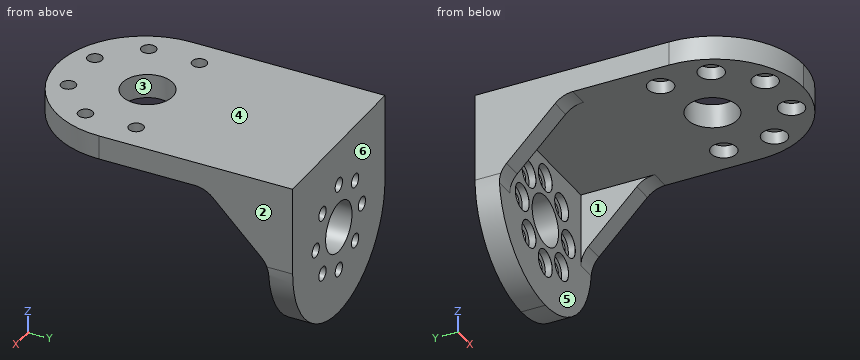
```python
from build123d import *

# Parameters (mm, degrees)
SKETCH1_W                      = 70
SKETCH1_H                      = 70
BOSS_EXTRUDE1_DEPTH            = 9.525
CBORE_FOR_M5_SBHCS1_AT_2_COUNT = 2
CBORE_FOR_M5_SBHCS1_AT_2_PITCH = 13.393920133
CBORE_FOR_M5_SBHCS1_AT_3_COUNT = 2
CBORE_FOR_M5_SBHCS1_AT_3_PITCH = 24.748737342
CBORE_FOR_M5_SBHCS1_AT_4_COUNT = 2
CBORE_FOR_M5_SBHCS1_AT_4_PITCH = 32.335783638
CBORE_FOR_M5_SBHCS1_AT_5_COUNT = 2
CBORE_FOR_M5_SBHCS1_AT_5_PITCH = 35
CBORE_FOR_M5_SBHCS1_AT_6_COUNT = 2
CBORE_FOR_M5_SBHCS1_AT_6_PITCH = 32.335783638
CBORE_FOR_M5_SBHCS1_AT_7_COUNT = 2
CBORE_FOR_M5_SBHCS1_AT_7_PITCH = 24.748737342
CBORE_FOR_M5_SBHCS1_AT_8_COUNT = 2
CBORE_FOR_M5_SBHCS1_AT_8_PITCH = 13.393920133
SKETCH5_R                      = 10
CUT_EXTRUDE1_DEPTH             = 51.405611047
SKETCH6_W                      = 70
SKETCH6_H                      = 102
BOSS_EXTRUDE2_DEPTH            = 9.525
CBORE_FOR_M5_SHCS1_D           = 5.8
CBORE_FOR_M5_SHCS1_CBORE_D     = 10
CBORE_FOR_M5_SHCS1_CBORE_DEPTH = 5
SKETCH7_R                      = 10
CUT_EXTRUDE3_DEPTH             = 9.525
BOSS_EXTRUDE3_DEPTH            = 8
FILLET1_R                      = 10
FILLET1_OF_MIRROR1_R           = 10
FILLET2_R                      = 35


with BuildPart() as part:
    # Sketch1 → Boss-Extrude1 (new body)
    with BuildSketch(Plane(origin=(0, 0, 0), x_dir=(1, 0, 0), z_dir=(0, 1, 0))):
        Rectangle(SKETCH1_W, SKETCH1_H)
    extrude(amount=BOSS_EXTRUDE1_DEPTH)

    # Sketch4 → CBORE for M5 SBHCS1 (revolve, cut)
    with BuildSketch(Plane(origin=(17.5, 0, 0), x_dir=(0, 0, -1), z_dir=(1, 0, 0))):
        Polygon((0, 0), (0, 9.525), (2.75, 9.525), (2.75, 2.75), (5.25, 2.75), (5.25, 0.025), (5.275, 0), align=None)
    cbore_for_m5_sbhcs1 = revolve(axis=Axis((17.5, -6.35, 0), (0, 1, 0)), mode=Mode.SUBTRACT)

    # CBORE for M5 SBHCS1 at 2: CBORE for M5 SBHCS1 ×2
    with Locations(*[Vector(-0.3826834323650897, 0, -0.9238795325112868) * (i * CBORE_FOR_M5_SBHCS1_AT_2_PITCH) for i in range(1, CBORE_FOR_M5_SBHCS1_AT_2_COUNT)]):
        add(cbore_for_m5_sbhcs1, mode=Mode.SUBTRACT)

    # CBORE for M5 SBHCS1 at 3: CBORE for M5 SBHCS1 ×2
    with Locations(*[Vector(-0.7071067811865476, 0, -0.7071067811865476) * (i * CBORE_FOR_M5_SBHCS1_AT_3_PITCH) for i in range(1, CBORE_FOR_M5_SBHCS1_AT_3_COUNT)]):
        add(cbore_for_m5_sbhcs1, mode=Mode.SUBTRACT)

    # CBORE for M5 SBHCS1 at 4: CBORE for M5 SBHCS1 ×2
    with Locations(*[Vector(-0.9238795325112867, 0, -0.38268343236508984) * (i * CBORE_FOR_M5_SBHCS1_AT_4_PITCH) for i in range(1, CBORE_FOR_M5_SBHCS1_AT_4_COUNT)]):
        add(cbore_for_m5_sbhcs1, mode=Mode.SUBTRACT)

    # CBORE for M5 SBHCS1 at 5: CBORE for M5 SBHCS1 ×2
    with Locations(*[(-i * CBORE_FOR_M5_SBHCS1_AT_5_PITCH, 0, 0) for i in range(1, CBORE_FOR_M5_SBHCS1_AT_5_COUNT)]):
        add(cbore_for_m5_sbhcs1, mode=Mode.SUBTRACT)

    # CBORE for M5 SBHCS1 at 6: CBORE for M5 SBHCS1 ×2
    with Locations(*[Vector(-0.9238795325112868, 0, 0.38268343236508967) * (i * CBORE_FOR_M5_SBHCS1_AT_6_PITCH) for i in range(1, CBORE_FOR_M5_SBHCS1_AT_6_COUNT)]):
        add(cbore_for_m5_sbhcs1, mode=Mode.SUBTRACT)

    # CBORE for M5 SBHCS1 at 7: CBORE for M5 SBHCS1 ×2
    with Locations(*[Vector(-0.7071067811865477, 0, 0.7071067811865475) * (i * CBORE_FOR_M5_SBHCS1_AT_7_PITCH) for i in range(1, CBORE_FOR_M5_SBHCS1_AT_7_COUNT)]):
        add(cbore_for_m5_sbhcs1, mode=Mode.SUBTRACT)

    # CBORE for M5 SBHCS1 at 8: CBORE for M5 SBHCS1 ×2
    with Locations(*[Vector(-0.3826834323650897, 0, 0.9238795325112868) * (i * CBORE_FOR_M5_SBHCS1_AT_8_PITCH) for i in range(1, CBORE_FOR_M5_SBHCS1_AT_8_COUNT)]):
        add(cbore_for_m5_sbhcs1, mode=Mode.SUBTRACT)

    # Sketch5 → Cut-Extrude1 (cut, through all)
    with BuildSketch(Plane.XZ):
        with Locations(Location((0, 0, 0), (0, 0, 270))):
            Circle(SKETCH5_R)
    extrude(amount=-CUT_EXTRUDE1_DEPTH, mode=Mode.SUBTRACT)

    # Sketch6 → Boss-Extrude2 (add)
    with BuildSketch(Plane.XY.offset(35)):
        with Locations((0, -51)):
            Rectangle(SKETCH6_W, SKETCH6_H)
    extrude(amount=-BOSS_EXTRUDE2_DEPTH)

    # CBORE for M5 SHCS1 (through all)
    with Locations(Plane(origin=(0, 0, 25.475), x_dir=(-1, 0, 0), z_dir=(0, 0, -1))):
        with Locations((-24, -58), (-24, -78), (-10, -92), (10, -92), (24, -78), (24, -58)):
            CounterBoreHole(CBORE_FOR_M5_SHCS1_D / 2, CBORE_FOR_M5_SHCS1_CBORE_D / 2, CBORE_FOR_M5_SHCS1_CBORE_DEPTH)

    # Sketch7 → Cut-Extrude3 (cut)
    with BuildSketch(Plane(origin=(0, 0, 25.475), x_dir=(-1, 0, 0), z_dir=(0, 0, -1))):
        with Locations((0, -66)):
            Circle(SKETCH7_R)
    extrude(amount=-CUT_EXTRUDE3_DEPTH, mode=Mode.SUBTRACT)

    # Sketch17 → Boss-Extrude3 (add)
    with BuildSketch(Plane.ZY.offset(35)):
        Polygon((25.475, 0), (25.475, -25), (0.475, 0), align=None)
    boss_extrude3 = extrude(amount=-BOSS_EXTRUDE3_DEPTH)

    # Fillet1
    fillet1_edges = [part.edges().sort_by_distance(p)[0] for p in [
        (-31, 0, 0.475),
        (-31, -25, 25.475),
    ]]
    fillet(fillet1_edges, radius=FILLET1_R)

    # Mirror1: Boss-Extrude3 across plane
    add(boss_extrude3.mirror(Plane(origin=(0, 0, 0), x_dir=(0, 0, 1), z_dir=(1, 0, 0))))

    # Fillet1 of Mirror1
    fillet1_of_mirror1_edges = [part.edges().sort_by_distance(p)[0] for p in [
        (31, 0, 0.475),
        (31, -25, 25.475),
    ]]
    fillet(fillet1_of_mirror1_edges, radius=FILLET1_OF_MIRROR1_R)

    # Fillet2
    fillet2_edges = [part.edges().sort_by_distance(p)[0] for p in [
        (-35, 4.7625, -35),
        (35, 4.7625, -35),
        (35, -102, 30.2375),
        (-35, -102, 30.2375),
    ]]
    fillet(fillet2_edges, radius=FILLET2_R - 0.0001)  # a hair under: the kernel refuses the full size


solid = part.part
```
Check sheet for the modelled part. Datum: model origin and axes. Units: mm. Face numbers are marked on the shaded views. A direction names the side the tool comes from. Round coordinates to 2 decimals unless told otherwise and drop trailing zeros. Loops run counter-clockwise (first coordinate to the right, second up) from the corner with the lowest first, then second, coordinate; pieces in that order, holes last. Notation, with made-up numbers: (35, 30) -> (65, 30) arc R32 ccw to (65, 63) -> close; hole circle Ø9 at (73.5, 81.25). An arc over 180 degrees is marked (long way). Write item = value, one per line. Start each with the question number.
1) Sectioned sample at B-B, the plane y = -12. Record the cut outline in (x, z) (3 decimals), plus the area to 3 significant figures.
2) Gauge pin test, flat ends, axial feed: pin 1 Ø3 at (x, y) = (-26, -79.5) entering from -Z (3 decimals); pin 2 Ø2 at (x, y) = (1.5, -5) entering from -Z (3 decimals); pin 3 Ø5 at (x, z) = (2, 16.5) entering from -Y. Record the tip position at first contact, or that the pin passes through.
3) Sectioned sample at A-A, the plane y = -78. Record the cut outline in (x, z) (3 decimals), plus the area to 3 significant figures.
4) Sectioned sample at C-C, the plane y = -34.5. Record the cut outline in (x, z) (3 decimals), plus the area to 3 significant figures.
5) Set-up check for the marked faces 1 and 2: record each of +Z, -Z, +X, -X, +Y, -Y from which the full face is reachable in a straight line by a thin tool's end or side.
6) Thickness scan on probe 1 along X at (y, z) = (6, 0); probe 2 along Y at (x, z) = (-5.5, 28.5) (3 decimals); probe 3 along Z at (x, y) = (13, 4.5). Record the ranges inside material, lowest first.
7) Release check for a two-part mould opening along Y. For the marked faces 3, 4, 5 and 6 record: released by +Y, released by -Y, zero draft, split by the parting line, or undercut.
Results are:
q1.outline = (-35, 12.475) -> (-27, 12.475) -> (-27, 25.475) -> (27, 25.475) -> (27, 12.475) -> (35, 12.475) -> (35, 35) -> (-35, 35) -> close
q1.area = 875 mm^2
q2.pin_1 = 30.475
q2.pin_2 = 25.475
q2.pin_3 = 2.75
q3.outline = (-33.227, 25.475) -> (-29, 25.475) -> (-29, 30.475) -> (-26.9, 30.475) -> (-26.9, 35) -> (-33.227, 35) -> close; (-21.1, 30.475) -> (-19, 30.475) -> (-19, 25.475) -> (19, 25.475) -> (19, 30.475) -> (21.1, 30.475) -> (21.1, 35) -> (-21.1, 35) -> close; (26.9, 30.475) -> (29, 30.475) -> (29, 25.475) -> (33.227, 25.475) -> (33.227, 35) -> (26.9, 35) -> close
q3.area = 480 mm^2
q4.outline = (-35, 25.475) -> (35, 25.475) -> (35, 35) -> (-35, 35) -> close
q4.area = 667 mm^2
q5.face_1 = -Z, -Y
q5.face_2 = +Z, -Z, +X, +Y, -Y
q6.probe_1 = -35 to -20.25, -14.75 to -10, 10 to 14.75, 20.25 to 35
q6.probe_2 = -101.565 to -94.179, -89.821 to -74.352, -57.648 to 9.525
q6.probe_3 = -32.5 to -15.05, -9.7 to 9.7, 15.05 to 35
q7.face_3 = undercut
q7.face_4 = zero draft
q7.face_5 = released by -Y
q7.face_6 = released by +Y
